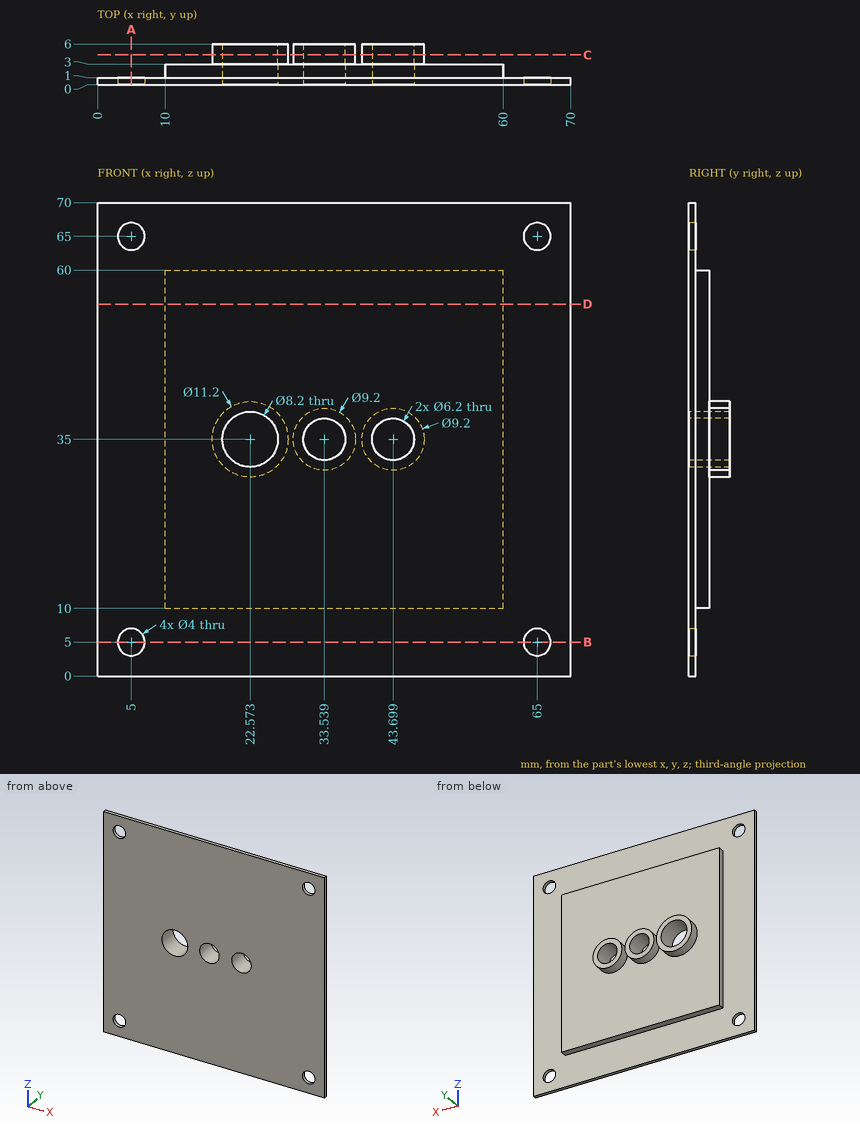
Study the drawing (mm; zero at the part's minimum x, y, z) and answer. Round coordinates to 2 decimals unless told otherwise and drop trailing zeros. Loops run counter-clockwise (first coordinate to the right, second up) from the corner with the lowest first, then second, coordinate; pieces in that order, holes last.
Q1. Section B-B, the plane z = 5 is taken. Determine the outline of the cut face in (x, y).
Q2. Find the intervals of material crossed by line 1 (X direction, y = 0.4, z = 5); line 2 (X direction, y = 1.2, z = 35), in increasing order.
Q3. Section A-A, the plane x = 5 is taken. Determine the outline of the cut face in (y, z).
Q4. Section D-D, the plane z = 55 is taken. Determine the outline of the cut face in (x, y), then the cut area to 3 significant figures.
Q5. Given pin 1 Ø1.5 at (y, z) = (3.5, 30.5) entering from -X; pin 2 Ø2 at (x, z) = (45, 10) entering from +Y; pin 3 Ø5.5 at (x, z) = (33.54, 35) entering from -Y; pin 4 Ø1.6 at (y, z) = (2, 41.5) entering from +X, each flat-ended and moving along its own axis, determine where each tip first touches the part or whether it passes through.
Q6. Section C-C, the plane y = 4.4 is taken. Determine the outline of the cut face in (x, z).
Completed:
1. outline: (0, 0) - (3, 0) - (3, 1) - (0, 1) - close; (7, 0) - (63, 0) - (63, 1) - (7, 1) - close; (67, 0) - (70, 0) - (70, 1) - (67, 1) - close
2. line 1: x = 0 to 3, 7 to 63, 67 to 70
2. line 2: x = 10 to 18.47, 26.67 to 30.44, 36.64 to 40.6, 46.8 to 60
3. outline: (0, 0) - (1, 0) - (1, 3) - (0, 3) - close; (0, 7) - (1, 7) - (1, 63) - (0, 63) - close; (0, 67) - (1, 67) - (1, 70) - (0, 70) - close
4. outline: (0, 0) - (70, 0) - (70, 1) - (60, 1) - (60, 3) - (10, 3) - (10, 1) - (0, 1) - close
4. area: 170 mm2
5. pin 1: stops at x = 10
5. pin 2: stops at y = 3
5. pin 3: passes through
5. pin 4: stops at x = 60
6. outline: circle Ø11.2 at (22.57, 35); circle Ø9.2 at (33.54, 35); circle Ø9.2 at (43.7, 35); hole circle Ø8.2 at (22.57, 35); hole circle Ø6.2 at (33.54, 35); hole circle Ø6.2 at (43.7, 35)
